Work out the finished part from the listing and answer in its coordinate system (mm). Face numbers are marked on the shaded views. Give positions to 0.01 mm unless a question says otherwise; leave off trailing zeros. Write each loop counter-clockwise with the first axis right and the second up, starting at its lowest first coordinate (ties: lowest second). Pieces come first, ordered by that corner, then holes. Notation, with made-up numbers: (66.25, 26) -> (93.25, 26) arc R11 cw to (93.25, 33) -> close; hole circle Ø9 at (-30.5, 32). An arc over 180 degrees is marked (long way). Use a Markdown table: item, result. Add a question column.
Q1. Each of these flat-tipped pins is pushed along its axis until it touches: pin 1 Ø1.5 at (x, y) = (-6.5, 11) entering from -Z; pin 2 Ø1.5 at (x, y) = (3, 6.5) entering from -Z; pin 3 Ø8 at (x, z) = (-6, -67.5) entering from +Y; pin 4 Ø9 at (x, z) = (0, -100) entering from -Y. Where does it stop, or does it pass through?
Q2. Section A-A, the plane x = 0 is taken. State how many separate pieces and enclosed holes the cut face has, plus the area to 3 significant figures.
Q3. Section C-C, the plane y = 5.5 is taken. Give the vertices of the cut face in (x, z).
Q4. Section B-B, the plane y = 12 is taken. Give the vertices of the cut face in (x, z), plus the area to 3 significant figures.
Q5. For a pull along X with two mould halves and no side action, classify the marked faces 1, 2, 3 and 4 as pulls with the +X half, pulls with the -X half, needs draft (parallel to the pull), parting line crosses it, or undercut.
Q6. Section D-D, the plane z = -21 is taken. Give the vertices of the cut face in (x, y), plus the area to 3 significant figures.
Q7. Consider line 1 (Z direction, x = 0, y = 5.5); line 2 (Z direction, x = 0, y = 12.75); line 3 (X direction, y = 7.25, z = -21). Determine where each line is inside the solid, lowest interval first.
Autodesk Inventor part; units mm, degrees
ref_plane "YZ Plane" through (0, 0, 0) normal (1, 0, 0) x (0, 1, 0)
ref_plane "XZ Plane" through (0, 0, 0) normal (0, 1, 0) x (-1, 0, 0)
ref_plane "XY Plane" through (0, 0, 0) normal (0, 0, 1) x (1, 0, 0)
sketch "Sketch1" plane through (0, 0, 0) normal (0, 1, 0) x (-1, 0, 0)
  circle A0 centre (0, 0) radius 10
  circle A1 centre (0, 0) radius 20
  line L0 (0, 0) -> (0, -100)
  circle A2 centre (0, -100) radius 10
  circle A3 centre (0, -100) radius 20
  line L1 (0, -100) -> (20, -100)
  line L2 (20, -100) -> (20, 0)
  line L3 (20, 0) -> (0, 0)
  line L4 (0, 0) -> (0, -100)
  line L5 (0, -100) -> (-20, -100)
  line L6 (-20, -100) -> (-20, 0)
  line L7 (-20, 0) -> (0, 0)
  line L8 (0, 0) -> (0, -100)
  point P0 (20, -100)
  dimension "d0" = 20
  dimension "d4" = 40
  dimension "d23" = 20
  dimension "d24" = 40
extrude "Extrusion1" add sketch "Sketch1" along normal blind 15 contours L3 A1 L0 A0 | A0 L7 A1 L3 | A0 L0 A1 L7 | L2 A3 L0 A1 | A1 L0 A3 L6 | L1 A2 L0 A3 | A3 L5 A2 L1 | A3 L0 A2 L5
shell "Shell2" thickness 7 removed faces 1 at (-15.2269, 15, -36.0766)
sketch "Sketch8" plane through (0, 15, 0) normal (0, 1, 0) x (1, 0, 0)
  line L0 (-13, 10.9545) -> (-13, 89.0455)
  arc A0 (-13, 89.0455) -> (13, 89.0455) centre (0, 100) ccw
  line L1 (13, 89.0455) -> (13, 10.9545)
  arc A1 (13, 10.9545) -> (-13, 10.9545) centre (0, 0) ccw
  arc A2 (-20, 0) -> (20, 0) centre (0, 0) ccw
  line L2 (20, 0) -> (20, 100)
  arc A3 (20, 100) -> (-20, 100) centre (0, 100) ccw
  line L3 (-20, 100) -> (-20, 0)
  circle A4 centre (0, 0) radius 10
  circle A5 centre (0, 100) radius 10
  circle A6 centre (0, 0) radius 5.5
  circle A7 centre (0, 100) radius 5.5
  dimension "d26" = 11
  dimension "d27" = 11
extrude "Extrusion8" add sketch "Sketch8" against normal blind 7.5 contours A4
sketch "Sketch9" plane through (0, 0, 0) normal (0, -1, 0) x (1, 0, 0)
  arc A0 (20, 0) -> (-20, 0) centre (0, 0) ccw
  line L0 (-20, -100) -> (-20, 0)
  arc A1 (-20, -100) -> (20, -100) centre (0, -100) ccw
  line L1 (20, 0) -> (20, -100)
  circle A2 centre (0, 0) radius 10
  circle A3 centre (0, -100) radius 10
  circle A4 centre (0, -100) radius 5.5
  dimension "d30" = 11
extrude "Extrusion9" add sketch "Sketch9" against normal blind 7.5 contours A3
chamfer "Chamfer1" distance 1 angle 45 2 edges at (10, 15, -100) (10, 0, 0)
chamfer "Chamfer2" distance 0.7 angle 45 2 edges at (-5.5, 15, 0) (-5.5, 0, -100)
properties part number "ramię_korby" material "ABS Plastic"
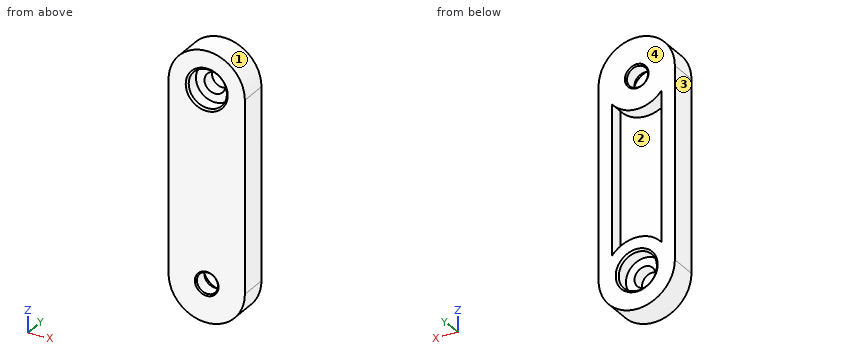
Result set:
| question | item | result |
|---|---|---|
| 1 | pin 1 | stops at z = -119.16 |
| 1 | pin 2 | stops at z = -119.87 |
| 1 | pin 3 | stops at y = 7 |
| 1 | pin 4 | passes through |
| 2 | separate pieces | 3 |
| 2 | enclosed holes | 0 |
| 2 | area | 1,100 mm2 |
| 3 | outline | (-20, -100) arc R20 ccw to (20, -100) -> (20, 0) arc R20 ccw to (-20, 0) -> close; hole circle Ø20 at (0, 0); hole circle Ø11 at (0, -100) |
| 4 | outline | (-20, -100) arc R20 ccw to (20, -100) -> (20, 0) arc R20 ccw to (-20, 0) -> close; hole (-13, -89.05) arc R17 cw to (13, -89.05) -> (13, -10.95) arc R17 cw to (-13, -10.95) -> close; hole circle Ø20 at (0, -100); hole circle Ø11 at (0, 0) |
| 4 | area | 3,040 mm2 |
| 5 | face 1 | parting line crosses it |
| 5 | face 2 | undercut |
| 5 | face 3 | pulls with the -X half |
| 5 | face 4 | needs draft |
| 6 | outline | (-20, 0) -> (20, 0) -> (20, 15) -> (13, 15) -> (13, 7) -> (-13, 7) -> (-13, 15) -> (-20, 15) -> close |
| 6 | area | 392 mm2 |
| 7 | line 1 | z = -120 to -105.5, -94.5 to -10, 10 to 20 |
| 7 | line 2 | z = -120 to -110, -90 to -83, -17 to -5.5, 5.5 to 20 |
| 7 | line 3 | x = -20 to -13, 13 to 20 |
